Part print with two shaded views. Sizes in mm from the minimum x, y, z corner. A direction names the side the tool comes from. Coordinates: 2 decimals unless noted, no trailing zeros. Loops run counter-clockwise (first coordinate to the right, second up) from the corner with the lowest first, then second, coordinate; pieces in that order, holes last. Notation, with made-up numbers: (66, 83) - (86, 83) arc R17 ccw to (86, 115) - close; hole circle Ø6 at (85.25, -8.75). An arc over 180 degrees is marked (long way). Answer as CSV lines item,"result".
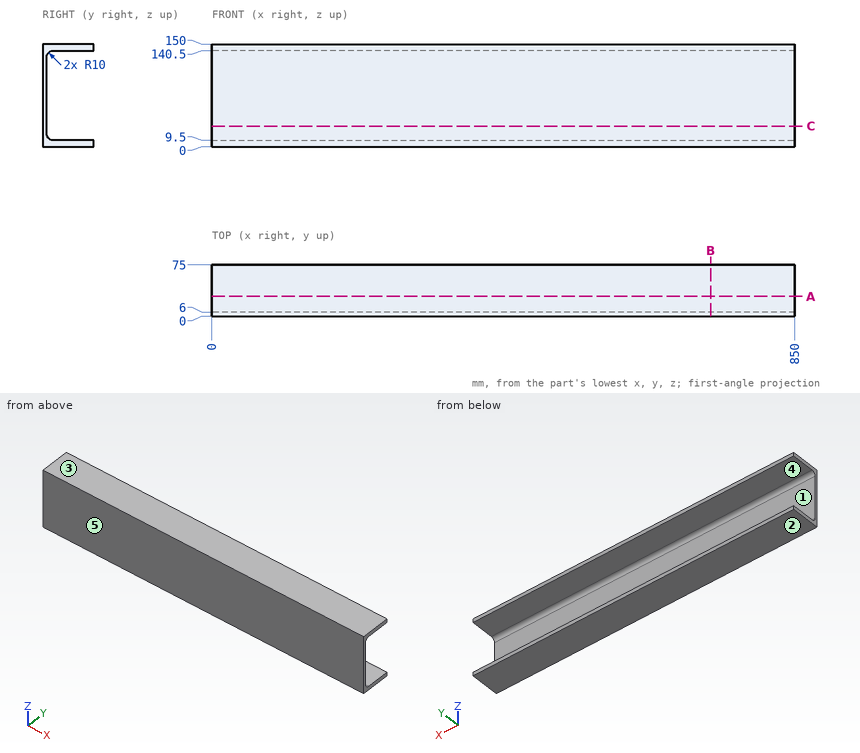
Q1. Saw through at B-B (x = 727.5). Give the cut face in (y, z), then the cut area to 3 significant figures.
Results:
outline,"(0, 0) - (75, 0) - (75, 9.5) - (16, 9.5) arc R10 cw to (6, 19.5) - (6, 130.5) arc R10 cw to (16, 140.5) - (75, 140.5) - (75, 150) - (0, 150) - close"
area,"2,250 mm^2"
Q2. Which spindle directions (+Z, -Z, +X, -X, +Y, -Y) get a long thin tool onto all of the face, cutting with end or side? Do the marked faces 1 and 2. Say none if no direction does.
Results:
face 1,"+X, -X, +Y"
face 2,"-Z, +X, -X, +Y, -Y"
Q3. Saw through at A-A (y = 29). Give the cut face in (x, z), then the cut area to 4 significant figures.
Results:
outline,"(0, 0) - (850, 0) - (850, 9.5) - (0, 9.5) - close; (0, 140.5) - (850, 140.5) - (850, 150) - (0, 150) - close"
area,"16,150 mm^2"
Q4. Saw through at C-C (z = 30). Give the cut face in (x, y), then the cut area to 3 significant figures.
Results:
outline,"(0, 0) - (850, 0) - (850, 6) - (0, 6) - close"
area,"5,100 mm^2"
Q5. Wall check: L1, parallel to Z at x = 349.5, y = 42; L2, parallel to Y at x = 733, z = 57.5; L3, parallel to Z at x = 176, y = 12.5. Give the ranges that are in metal, low to high.
Results:
L1,"z = 0 to 9.5, 140.5 to 150"
L2,"y = 0 to 6"
L3,"z = 0 to 10.13, 139.87 to 150"
Q6. Flat gauge pin, fed straight in: pin 1 (5 mm diameter, centred on x = 618.5, z = 97, fed in from +Y). Where does the tip first touch, or does it go through?
Results:
pin 1,"stops at y = 6"
Q7. Two-plate mould, pull along Z, no slides. Class the marked faces 3, 4 and 5: released by +Z, released by -Z, zero draft, split by the parting line, or undercut.
Results:
face 3,"released by +Z"
face 4,"undercut"
face 5,"zero draft"
